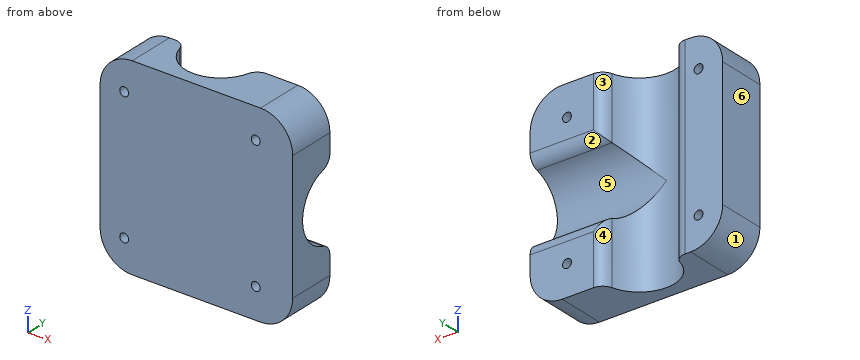
from build123d import *

# Parameters (mm, degrees)
SKETCH1_W           = 19.05
SKETCH1_H           = 76.2
SKETCH1_R           = 1.75
SKETCH1_W_2         = 29.21
SKETCH1_H_2         = 24.13
SKETCH1_H_3         = 27.94
BOSS_EXTRUDE2_DEPTH = 19.05
SKETCH3_R           = 13.97
CUT_EXTRUDE2_DEPTH  = 77.2
CUT_EXTRUDE3_REACH  = 78.2
SKETCH4_R           = 13.97
FILLET1_R           = 4.7625
FILLET2_R           = 12.7


with BuildPart() as part:
    # Sketch1 → Boss-Extrude2 (new body)
    with BuildSketch(Plane(origin=(0, 0, 0), x_dir=(1, 0, 0), z_dir=(0, 1, 0))):
        with Locations((9.525, 38.1)):
            Rectangle(SKETCH1_W, SKETCH1_H)
        with Locations((9.525, 12.065)):
            Circle(SKETCH1_R, mode=Mode.SUBTRACT)
        with Locations((9.525, 64.135)):
            Circle(SKETCH1_R, mode=Mode.SUBTRACT)
        Polygon((19.05, 76.2), (19.05, 0), (46.99, 0), (46.99, 24.13), (46.99, 52.07), (46.99, 76.2), align=None)
        with Locations((61.595, 64.135)):
            Rectangle(SKETCH1_W_2, SKETCH1_H_2)
        with Locations((61.595, 64.135)):
            Circle(SKETCH1_R, mode=Mode.SUBTRACT)
        with Locations((61.595, 38.1)):
            Rectangle(SKETCH1_W_2, SKETCH1_H_3)
        with Locations((61.595, 12.065)):
            Rectangle(SKETCH1_W_2, SKETCH1_H_2)
        with Locations((61.595, 12.065)):
            Circle(SKETCH1_R, mode=Mode.SUBTRACT)
    extrude(amount=BOSS_EXTRUDE2_DEPTH)

    # Sketch3 → Cut-Extrude2 (cut, through all)
    with BuildSketch(Plane.XY):
        with Locations((33.02, 19.05)):
            Circle(SKETCH3_R)
    extrude(amount=-CUT_EXTRUDE2_DEPTH, mode=Mode.SUBTRACT)

    # Sketch4 → Cut-Extrude3 (cut, up to next)
    with BuildSketch(Plane(origin=(76.2, 0, 0), x_dir=(0, 0, -1), z_dir=(1, 0, 0)), mode=Mode.PRIVATE) as cut_extrude3_sk1:
        with Locations((38.1, 19.05)):
            Circle(SKETCH4_R)
    cut_extrude3_tool1 = extrude(cut_extrude3_sk1.sketch, amount=-CUT_EXTRUDE3_REACH, mode=Mode.PRIVATE) & part.part
    add(cut_extrude3_tool1.solids().sort_by_distance((76.2, 19.05, -38.1))[0], mode=Mode.SUBTRACT)

    # Fillet1
    fillet1_edges = [part.edges().sort_by_distance(p)[0] for p in [
        (46.99, 19.05, -12.065),
        (61.595, 19.05, -24.13),
        (61.595, 19.05, -52.07),
        (46.99, 19.05, -64.135),
        (19.05, 19.05, -38.1),
    ]]
    fillet(fillet1_edges, radius=FILLET1_R)

    # Fillet2
    fillet2_edges = [part.edges().sort_by_distance(p)[0] for p in [
        (0, 9.525, 0),
        (0, 9.525, -76.2),
        (76.2, 9.525, -76.2),
        (76.2, 9.525, 0),
    ]]
    fillet(fillet2_edges, radius=FILLET2_R)


solid = part.part
Can you work these out from the model? Positions are in its coordinate system, mm. Face numbers are marked on the shaded views. A direction names the side the tool comes from. Give positions to 0.01 mm unless a question says otherwise; leave off trailing zeros. Write each loop counter-clockwise with the first axis right and the second up, starting at its lowest first coordinate (ties: lowest second). Pieces come first, ordered by that corner, then holes. Notation, with made-up numbers: (47.5, 87) -> (100.5, 87) arc R31 cw to (100.5, 113) -> close; hole circle Ø7 at (-9, 52.5). An arc over 180 degrees is marked (long way). Answer as a JSON object with one key per item and string values. Group by question number.
Item 1: For the marked faces 4, 5 and 6, which set-ups out of +Z, -Z, +X, -X, +Y, -Y let a thin tool reach every point of the face, with its end or its side?
Item 2: Suppose I cut it at D-D (y = 3). Please give me the cut outline in (x, z) (3 decimals).
Item 3: Please list where these lines run through material, in increasing order: line 1 (Z direction, x = 61.5, y = 16); line 2 (Z direction, x = 10, y = 4.25); line 3 (X direction, y = 16, z = -22.5). Write a range as [from, to].
Item 4: We'd pull the mould along Z, two halves only. Please class the marked faces 1, 2 and 3: +Z half, -Z half, draft (parallel to the pull), parting line (faces both ways), or undercut.
Item 5: I'm going to push flat-ended pins straight in: P1, Ø2, axis at x = 23, z = -18.5, coming from the +Y side; P2, Ø4.5, axis at x = 61.595, z = -12.065, coming from the +Y side; P3, Ø10, axis at x = 60, z = -37, coming from the +Y side. Where does each tip first touch, or does it pass through?
Item 6: Suppose I cut it at B-B (y = 13). Please give me the cut outline in (x, z) (3 decimals).
Findings:
{
 "1": {"face 4": "+Z, -Z, +Y", "face 5": "+X, +Y", "face 6": "+Z, -Z, -X, +Y, -Y"},
 "2": {"outline": "(0, -63.5) arc R12.7 ccw to (12.7, -76.2) -> (63.5, -76.2) arc R12.7 ccw to (76.2, -63.5) -> (76.2, -12.7) arc R12.7 ccw to (63.5, 0) -> (12.7, 0) arc R12.7 ccw to (0, -12.7) -> close; hole circle Ø3.5 at (9.525, -64.135); hole circle Ø3.5 at (9.525, -12.065); hole circle Ø3.5 at (61.595, -64.135); hole circle Ø3.5 at (61.595, -12.065)"},
 "3": {"line 1": "z = [-76.2, -65.88], [-62.39, -51.77], [-24.43, -13.81], [-10.32, 0]", "line 2": "z = [-75.91, -65.82], [-62.45, -13.75], [-10.38, -0.29]", "line 3": "x = [0, 19.35], [46.69, 76.2]"},
 "4": {"face 1": "-Z half", "face 2": "undercut", "face 3": "draft"},
 "5": {"P1": "stops at y = 10.46", "P2": "stops at y = 19.05", "P3": "stops at y = 6.48"},
 "6": {"outline": "(0, -63.5) arc R12.7 ccw to (12.7, -76.2) -> (20.428, -76.2) -> (20.428, 0) -> (12.7, 0) arc R12.7 ccw to (0, -12.7) -> close; (45.612, -76.2) -> (63.5, -76.2) arc R12.7 ccw to (76.2, -63.5) -> (76.2, -50.692) -> (45.612, -50.692) -> close; (45.612, -25.508) -> (76.2, -25.508) -> (76.2, -12.7) arc R12.7 ccw to (63.5, 0) -> (45.612, 0) -> close; hole circle Ø3.5 at (9.525, -64.135); hole circle Ø3.5 at (9.525, -12.065); hole circle Ø3.5 at (61.595, -64.135); hole circle Ø3.5 at (61.595, -12.065)"}
}
